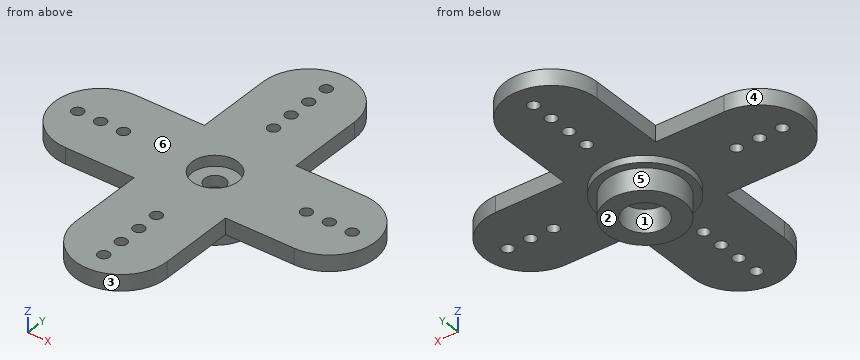
Autodesk Inventor part; units mm, degrees
ref_plane "YZ Plane" through (0, 0, 0) normal (1, 0, 0) x (0, 1, 0)
ref_plane "XZ Plane" through (0, 0, 0) normal (0, 1, 0) x (-1, 0, 0)
ref_plane "XY Plane" through (0, 0, 0) normal (0, 0, 1) x (1, 0, 0)
sketch "Sketch1" plane through (0, 0, 0) normal (1, 0, 0) x (0, 1, 0)
  line L0 (0, 0) -> (6, 0)
  line L1 (6, 0) -> (6, -2.85)
  line L2 (6, -2.85) -> (0, -2.85)
  line L3 (0, -2.85) -> (0, 0)
  line L4 (0, 0) -> (3, 0)
  line L5 (3, 0) -> (3, -1.4)
  line L6 (3, -1.4) -> (0, -1.4)
  line L7 (0, -1.4) -> (0, 0)
  line L8 (0, -1.4) -> (1.35, -1.4)
  line L9 (1.35, -1.4) -> (1.35, -2.85)
  line L10 (1.35, -2.85) -> (0, -2.85)
  line L11 (0, -2.85) -> (0, -1.4)
  line L12 (0, -2.85) -> (5, -2.85)
  line L13 (5, -2.85) -> (5, -5.85)
  line L14 (5, -5.85) -> (0, -5.85)
  line L15 (0, -5.85) -> (0, -2.85)
  line L16 (0, -2.85) -> (2.75, -2.85)
  line L17 (2.75, -2.85) -> (2.75, -5.85)
  line L18 (2.75, -5.85) -> (0, -5.85)
  line L19 (0, -5.85) -> (0, -2.85)
  point P0 (1.5, 0)
  point P1 (1.5, -1.4)
  dimension "d0" = 6
  dimension "d1" = 2.85
  dimension "d2" = 3
  dimension "d3" = 1.4
  dimension "d4" = 1.35
  dimension "d5" = 1.45
  dimension "d6" = 5
  dimension "d7" = 3
  dimension "d8" = 2.75
  dimension "d9" = 3
revolve "Revolution1" add sketch "Sketch1" angle 360 about axis through (0, 0, -2.85) along (0, 0, 1) contours L0 L1 L2 L9 L6 L5 | L13 L14 L17 L2
sketch "Sketch2" plane through (0, 0, 0) normal (0, 0, 1) x (1, 0, 0)
  point P0 (0, 0)
sketch "Sketch3" plane through (0, 0, 0) normal (0, 0, 1) x (1, 0, 0)
  circle A0 centre (0, 16) radius 6
  circle A1 centre (-15, 0) radius 6
  circle A2 centre (0, -16) radius 6
  circle A3 centre (15, 0) radius 6
  line L0 (-6, 16) -> (-6, -16)
  line L1 (6, 16) -> (6, -16)
  line L2 (-15, 6) -> (15, 6)
  line L3 (-15, -6) -> (15, -6)
  circle A4 centre (0, 10) radius 0.75
  circle A5 centre (0, 13) radius 0.75
  circle A6 centre (0, 16) radius 0.75
  circle A7 centre (0, 19) radius 0.75
  circle A8 centre (0, -19) radius 0.75
  circle A9 centre (0, -16) radius 0.75
  circle A10 centre (0, -13) radius 0.75
  circle A11 centre (0, -10) radius 0.75
  circle A12 centre (-12, 0) radius 0.75
  circle A13 centre (-15, 0) radius 0.75
  circle A14 centre (-18, 0) radius 0.75
  circle A15 centre (12, 0) radius 0.75
  circle A16 centre (15, 0) radius 0.75
  circle A17 centre (18, 0) radius 0.75
  point P0 (0, 0)
  point P1 (-6, 6)
  point P2 (-6, -6)
  point P3 (6, -6)
  point P4 (6, 6)
  dimension "d11" = 12
  dimension "d12" = 16
  dimension "d13" = 12
  dimension "d14" = 15
  dimension "d15" = 12
  dimension "d16" = 16
  dimension "d17" = 12
  dimension "d18" = 15
  dimension "d19" = 1.5
  dimension "d20" = 1.5
  dimension "d21" = 1.5
  dimension "d22" = 1.5
  dimension "d23" = 10
  dimension "d24" = 13
  dimension "d25" = 16
  dimension "d26" = 19
  dimension "d27" = 1.5
  dimension "d28" = 1.5
  dimension "d29" = 1.5
  dimension "d30" = 1.5
  dimension "d31" = 10
  dimension "d32" = 13
  dimension "d33" = 16
  dimension "d34" = 19
  dimension "d35" = 1.5
  dimension "d36" = 1.5
  dimension "d37" = 1.5
  dimension "d38" = 12
  dimension "d39" = 15
  dimension "d40" = 18
  dimension "d41" = 1.5
  dimension "d42" = 1.5
  dimension "d43" = 1.5
  dimension "d44" = 18
  dimension "d45" = 15
  dimension "d46" = 12
extrude "Extrusion1" add sketch "Sketch3" against normal blind 2.1 contours A0 A4 | L1 L2 L0 A0 A4 | L2 A3 L3 L1 | L1 L3 L0 L2 | L0 L3 A1 L2 | L1 A2 A11 L0 L3 | A3 | A1 | A2 A11 picked at (-2.215, 14.0731) picked at (-2.215, -14.0731)
revolve "Revolution2" cut sketch "Sketch1" angle 360 about axis through (0, 0, -2.85) along (0, 0, 1) contours L0 L5 L6 L3 | L6 L9 L2 L3 | L2 L17 L14 L15
sketch "Sketch4" plane through (0, 0, -2.85) normal (0, 0, -1) x (-1, 0, 0)
  circle A0 centre (0, 0) radius 6
  circle A1 centre (0, 0) radius 1.35
  circle A2 centre (0, 0) radius 5
extrude "Extrusion2" add sketch "Sketch4" along normal blind 0.15 contours A0
properties part number "Standar Servo Horn - Red"
The model under review builds one solid part; all positions refer to its coordinate system, in mm. Face numbers are marked on the shaded views. A direction names the side the tool comes from. Round coordinates to 2 decimals unless told otherwise and drop trailing zeros. Loops run counter-clockwise (first coordinate to the right, second up) from the corner with the lowest first, then second, coordinate; pieces in that order, holes last. Notation, with made-up numbers: (-14.5, 24.25) -> (6.5, 24.25) arc R6 ccw to (6.5, 32.25) -> close; hole circle Ø6 at (22, 67). An arc over 180 degrees is marked (long way). Answer as CSV lines item,"result".
1) To check wall thickness, follow line 1 along Y through (x, z) = (12, -0.4); line 2 along X through (y, z) = (0, -4.35); line 3 along Y through (x, z) = (4, -4.4). State the ranges of each line that lie inside material, in increasing order. Write a range as from..to.
Geometry results:
line 1,"y = -6..-0.75, 0.75..6"
line 2,"x = -5..-2.75, 2.75..5"
line 3,"y = -3..3"
2) Tool access review of the marked faces 5 and 6: name each direction out of +Z, -Z, +X, -X, +Y, -Y from which nothing blocks a thin tool from reaching the whole face with its end or side.
Geometry results:
face 5,"-Z"
face 6,"+Z, +X, -X, +Y, -Y"
3) Draft analysis for pull direction Y (two halves, no side actions). For the marked faces 1, 2, 3 and 4, state which applies: pulls with the +Y half, pulls with the -Y half, needs draft (parallel to the pull), parting line crosses it, or undercut.
Geometry results:
face 1,"undercut"
face 2,"needs draft"
face 3,"pulls with the -Y half"
face 4,"parting line crosses it"
4) Add section B-B on z = -0.65. State how many separate pieces and enclosed holes the cut face has, plus the area to 3 significant figures.
Geometry results:
separate pieces,"1"
enclosed holes,"15"
area,"773 mm²"
5) Add section C-C on x = -18. Write out the cut boundary in (y, z), plus the area to 3 significant figures.
Geometry results:
outline,"(-5.2, -2.1) -> (-0.75, -2.1) -> (-0.75, 0) -> (-5.2, 0) -> close; (0.75, -2.1) -> (5.2, -2.1) -> (5.2, 0) -> (0.75, 0) -> close"
area,"18.7 mm²"
6) Add section D-D on z = -4.55. Write out the cut boundary in (x, y), plus the area to 3 significant figures.
Geometry results:
outline,"circle Ø10 at (0, 0); hole circle Ø5.5 at (0, 0)"
area,"54.8 mm²"
7) Add section A-A on y = 13. Write out the cut boundary in (x, z), plus the area to 4 significant figures.
Geometry results:
outline,"(-6, -2.1) -> (-0.75, -2.1) -> (-0.75, 0) -> (-6, 0) -> close; (0.75, -2.1) -> (6, -2.1) -> (6, 0) -> (0.75, 0) -> close"
area,"22.05 mm²"
8) For P1, Ø1.5, axis at x = -13.5, z = -2, coming from the +Y side; P2, Ø0.6, axis at x = 12, z = -1.5, coming from the -Y side; P3, Ø1.7, axis at x = 0, y = -16, coming from the -Z side; P4, Ø1.2, axis at x = -12, y = 0, coming from the -Z side, all flat-tipped, find the tip position at first contact; note any pin that passes through.
Geometry results:
P1,"stops at y = 6"
P2,"stops at y = -6"
P3,"stops at z = -2.1"
P4,"passes through"
